Can you work these out from the drawing? Everything is in mm from the part's minimum corner. A direction names the side the tool comes from. Give positions to 0.01 mm unless a question says otherwise; leave off trailing zeros. Write each loop counter-clockwise with the first axis right and the second up, starting at its lowest first coordinate (ties: lowest second). Pieces come first, ordered by that corner, then holes. Notation, with made-up numbers: (-14, 64.25) -> (3, 64.25) arc R7 cw to (3, 73.25) -> close; hole circle Ø8 at (88, -39). An arc over 180 degrees is marked (long way). Write item = value, one per line. Start each with the question number.
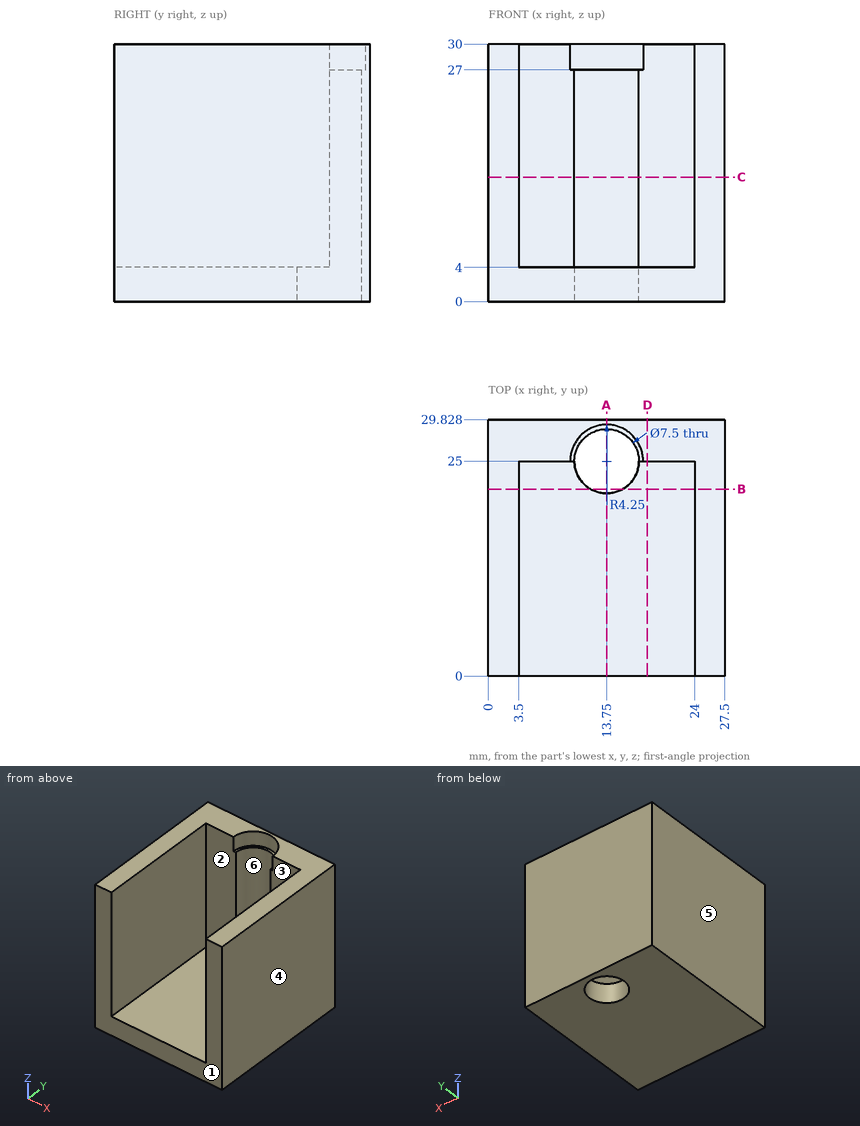
(1) I'm going to push flat-ended pins straight in: pin 1 (12 mm diameter, centred on x = 8, y = 3.5, fed in from +Z); pin 2 (10 mm diameter, centred on x = 13.5, z = 26, fed in from -Y); pin 3 (6 mm diameter, centred on x = 7.5, y = 13, fed in from +Z). Where does each tip first touch, or does it pass through?
(2) Imagine slicing it at A-A (x = 13.75). Please give me the cut outline in (y, z), then the cut area to 3 significant figures.
(3) Imagine slicing it at C-C (z = 14.5). Please give me the cut outline in (x, y), then the cut area to 3 significant figures.
(4) On a 3-axis mill with a long thin cutter (end or side, diameter ignored), from which of +Z, -Z, +X, -X, +Y, -Y can I reach the whole of each face in a straight line? I mean the marked faces 1 and 2. Say none if no direction works.
(5) Imagine slicing it at B-B (y = 21.75). Please give me the cut outline in (x, z), then the cut area to 3 significant figures.
(6) Imagine slicing it at D-D (x = 18.5). Please give me the cut outline in (y, z), then the cut area to 3 significant figures.
(7) If I drill on line 1 along X through (y, z) = (13.25, 20.5); line 2 along Z through (x, y) = (15.5, 5.25); line 3 along Y through (x, z) = (23.75, 12), over which ranges is the centre line in solid material (lowest first)? Write a range as from..to.
(8) We'd pull the mould along X, two halves only. Please class the marked faces 3, 4, 5 and 6: released by +X, released by -X, zero draft, split by the parting line, or undercut.
Answers below:
q1.pin_1 = 30
q1.pin_2 = 25
q1.pin_3 = 4
q2.outline = (0, 0) -> (21.25, 0) -> (21.25, 4) -> (0, 4) -> close; (28.75, 0) -> (29.83, 0) -> (29.83, 30) -> (29.25, 30) -> (29.25, 27) -> (28.75, 27) -> close
q2.area = 116 mm^2
q3.outline = (0, 0) -> (3.5, 0) -> (3.5, 25) -> (10, 25) arc R3.75 cw to (17.5, 25) -> (24, 25) -> (24, 0) -> (27.5, 0) -> (27.5, 29.83) -> (0, 29.83) -> close
q3.area = 286 mm^2
q4.face_1 = +Z, -Z, +X, -X, -Y
q4.face_2 = +Z, -Y
q5.outline = (0, 0) -> (11.88, 0) -> (11.88, 4) -> (3.5, 4) -> (3.5, 30) -> (0, 30) -> close; (15.62, 0) -> (27.5, 0) -> (27.5, 30) -> (24, 30) -> (24, 4) -> (15.62, 4) -> close
q5.area = 277 mm^2
q6.outline = (0, 0) -> (29.83, 0) -> (29.83, 30) -> (25, 30) -> (25, 4) -> (0, 4) -> close
q6.area = 245 mm^2
q7.line_1 = 0..3.5, 24..27.5
q7.line_2 = 0..4
q7.line_3 = 25..29.83
q8.face_3 = undercut
q8.face_4 = released by +X
q8.face_5 = released by -X
q8.face_6 = undercut
